Source: CAD feature listing. Evaluate the final solid. Frame: model axes, mm. Coordinates: 2 decimals unless noted, no trailing zeros. Write each loop counter-clockwise with the first axis right and the second up, starting at its lowest first coordinate (ties: lowest second). Pieces come first, ordered by that corner, then holes. Notation, with made-up numbers: (26, 34.5) - (67, 34.5) arc R13 cw to (67, 43.5) - close; hole circle Ø5 at (36.5, 45.25). An arc over 180 degrees is marked (long way). One line per item, written item: value.
from build123d import *

# Parameters (mm, degrees)
CROQUIS1_W              = 42.5
CROQUIS1_H              = 30
CROQUIS1_R              = 1.5
SALIENTE_EXTRUIR1_DEPTH = 3


with BuildPart() as part:
    # Croquis1 → Saliente-Extruir1 (new body)
    with BuildSketch(Plane.XY):
        with Locations((21.25, 15)):
            Rectangle(CROQUIS1_W, CROQUIS1_H)
        with Locations((6, 25)):
            Circle(CROQUIS1_R, mode=Mode.SUBTRACT)
        with Locations(Location((6, 5, 0), (0, 0, 180))):
            Circle(CROQUIS1_R, mode=Mode.SUBTRACT)
        with Locations((37.5, 15)):
            Circle(CROQUIS1_R, mode=Mode.SUBTRACT)
        with Locations((30.2, 15)):
            Circle(CROQUIS1_R, mode=Mode.SUBTRACT)
    extrude(amount=SALIENTE_EXTRUIR1_DEPTH)


solid = part.part
1) Contact query for a flat-ended pin moving along its axis: P1, Ø2.5, axis at x = 30.2, y = 15, coming from the -Z side. Output: stop coordinate, or through.
Values found:
P1: through
2) Section query B-B on x = 37.5. Output: boundary loops of the cut face in (y, z).
Values found:
outline: (0, 0) - (13.5, 0) - (13.5, 3) - (0, 3) - close; (16.5, 0) - (30, 0) - (30, 3) - (16.5, 3) - close
3) Section query A-A on y = 15. Output: boundary loops of the cut face in (x, z).
Values found:
outline: (0, 0) - (28.7, 0) - (28.7, 3) - (0, 3) - close; (31.7, 0) - (36, 0) - (36, 3) - (31.7, 3) - close; (39, 0) - (42.5, 0) - (42.5, 3) - (39, 3) - close
4) Material intervals for line 1 (Y direction, x = 6, z = 1.05); line 2 (X direction, y = 13.75, z = 1.5); line 3 (Y direction, x = 30.2, z = 1.5), sorted ascending.
Values found:
line 1: 0 to 3.5, 6.5 to 23.5, 26.5 to 30
line 2: 0 to 29.37, 31.03 to 36.67, 38.33 to 42.5
line 3: 0 to 13.5, 16.5 to 30
5) Section query C-C on z = 2.25. Output: boundary loops of the cut face in (x, y).
Values found:
outline: (0, 0) - (42.5, 0) - (42.5, 30) - (0, 30) - close; hole circle Ø3 at (6, 5); hole circle Ø3 at (6, 25); hole circle Ø3 at (30.2, 15); hole circle Ø3 at (37.5, 15)
6) Draft query along Y for faces 1 (the cylindrical face through (7.11, 3.99, 1.48)), 2 (the flat face through (21, 15, 3)), 3 (the flat face through (21, 30, 1)). Return one class per face: released by +Y, released by -Y, zero draft, split by the parting line, or undercut.
Values found:
face 1: undercut
face 2: zero draft
face 3: released by +Y
7) Section query D-D on y = 5. Output: boundary loops of the cut face in (x, z), then the cut area to 4 significant figures.
Values found:
outline: (0, 0) - (4.5, 0) - (4.5, 3) - (0, 3) - close; (7.5, 0) - (42.5, 0) - (42.5, 3) - (7.5, 3) - close
area: 118.5 mm2
